Verification items for the finished model (mm, model axes). A direction names the side the tool comes from. Coordinates: 2 decimals unless noted, no trailing zeros. Loops run counter-clockwise (first coordinate to the right, second up) from the corner with the lowest first, then second, coordinate; pieces in that order, holes last. Notation, with made-up numbers: (46.25, 28) -> (63.25, 28) arc R19 ccw to (63.25, 34) -> close; hole circle Ø11 at (57.25, -8.75). An arc over 180 degrees is marked (long way). Answer as a JSON object with one key per item and string values. Group by question number.
Q1. Cross-section at A-A on z = 9.25. Record the boundary of the cut face in (x, y), and give its area (3 significant figures).
Q2. Release check for a two-part mould opening along X. For faces 6 (the cylindrical face through (53.496, 6.926, -4.93)), 7 (the flat face through (27, 1, 0.81)), 8 (the cylindrical face through (65.2, 0.57, 0.41)), 9 (the flat face through (22, 7, 15.82)) record: released by +X, released by -X, zero draft, split by the parting line, or undercut.
Q3. Gauge pin test, flat ends, axial feed: pin 1 Ø3 at (x, y) = (58, 5.5) entering from +Z; pin 2 Ø3 at (x, z) = (47.5, 7.5) entering from -Y; pin 3 Ø3.5 at (x, z) = (25.5, 4.5) entering from +Y. Record the tip position at first contact, or that the pin passes through.
Q4. Cross-section at D-D on x = 18.5. Record the boundary of the cut face in (y, z), and give its area (3 significant figures).
Q5. Cross-section at C-C on z = -5.5. Record the boundary of the cut face in (x, y).
Q6. Scan lines: L1, parallel to X at y = 13, z = 8.25; L2, parallel to Y at x = 5.1, z = 1.5; L3, parallel to X at y = 7.5, z = -1.25. Record each from-to range of solid material in increasing order.
Q7. Set-up check for faces 1 (the cylindrical face through (34.682, 5.914, -4.93)), 2 (the flat face through (58, 12.2, 4)), 3 (the flat face through (50, 2, 4)), 4 (the flat face through (8, 7, 7.92)), 5 (the flat face through (49, 13, 0.81)): record each of +Z, -Z, +X, -X, +Y, -Y from which the full face is reachable in a straight line by a thin tool's end or side.
Q8. Cross-section at B-B on x = 49.55. Record the boundary of the cut face in (y, z).
Autodesk Inventor part; units mm, degrees
ref_plane "YZ Plane" through (0, 0, 0) normal (1, 0, 0) x (0, 1, 0)
ref_plane "XZ Plane" through (0, 0, 0) normal (0, 1, 0) x (-1, 0, 0)
ref_plane "XY Plane" through (0, 0, 0) normal (0, 0, 1) x (1, 0, 0)
sketch "Sketch1" plane through (0, 0, 0) normal (0, 0, 1) x (1, 0, 0)
  line L0 (0, 0) -> (65.8, 0)
  line L1 (65.8, 0) -> (65.8, 14.2)
  line L2 (65.8, 14.2) -> (0, 14.2)
  line L3 (0, 14.2) -> (0, 0)
  dimension "d0" = 65.8
  dimension "d1" = 14.2
extrude "Extrusion1" add sketch "Sketch1" along normal blind 0.81
fillet "Fillet1" radius 2 4 edges at (0, 14.2, 0.405) (65.8, 14.2, 0.405) (65.8, 0, 0.405) (0, 0, 0.405)
sketch "Sketch2" plane through (0, 0, 0.81) normal (0, 0, 1) x (1, 0, 0)
  circle A0 centre (5.1, 7.1) radius 5.1
  line L0 (0, 12.2) -> (0, 2)
  circle A1 centre (60.7, 7.1) radius 5.1
  line L1 (65.8, 2) -> (65.8, 12.2)
  line L2 (5.1, 12.2) -> (60.7, 12.2)
  line L3 (60.7, 2) -> (5.1, 2)
  point P0 (0, 0)
  point P1 (0, 7.1)
  dimension "d5" = 10.2
  dimension "d6" = 10.2
extrude "Extrusion2" add sketch "Sketch2" along normal blind 7.11
sketch "Sketch3" plane through (0, 0, 7.92) normal (0, 0, 1) x (1, 0, 0)
  line L0 (2, 0) -> (63.8, 0)
  line L1 (32.9, 0) -> (32.9, 14.2) construction
  line L2 (63.8, 14.2) -> (2, 14.2)
  circle A0 centre (5.1, 7.1) radius 2.4
  circle A1 centre (60.7, 7.1) radius 2.4
  line L3 (5.1, 7.1) -> (60.7, 7.1) construction
  point P0 (0, 0)
  dimension "d9" = 4.8
  dimension "d10" = 4.8
  dimension "d12" = 27.8
  dimension "d13" = 27.8
  dimension "d14" = 7.1
extrude "Extrusion3" cut sketch "Sketch3" against normal through all
sketch "Sketch4" plane through (0, 0, 7.92) normal (0, 0, 1) x (1, 0, 0)
  line L0 (63.8, 14.2) -> (2, 14.2)
  line L1 (32.9, 14.2) -> (32.9, 0) construction
  line L2 (2, 0) -> (63.8, 0)
  line L3 (31.9, 14.2) -> (33.9, 14.2)
  line L4 (33.9, 14.2) -> (33.9, 0)
  line L5 (33.9, 0) -> (31.9, 0)
  line L6 (31.9, 0) -> (31.9, 14.2)
  line L7 (20.8, 14.2) -> (22.8, 14.2)
  line L8 (22.8, 14.2) -> (22.8, 0)
  line L9 (22.8, 0) -> (20.8, 0)
  line L10 (20.8, 0) -> (20.8, 14.2)
  line L11 (11.7, 0) -> (9.7, 0)
  line L12 (9.7, 0) -> (9.7, 14.2)
  line L13 (9.7, 14.2) -> (11.7, 14.2)
  line L14 (11.7, 14.2) -> (11.7, 0)
  line L15 (43, 14.2) -> (45, 14.2)
  line L16 (45, 14.2) -> (45, 0)
  line L17 (45, 0) -> (43, 0)
  line L18 (43, 0) -> (43, 14.2)
  line L19 (54.1, 0) -> (56.1, 0)
  line L20 (56.1, 0) -> (56.1, 14.2)
  line L21 (56.1, 14.2) -> (54.1, 14.2)
  line L22 (54.1, 14.2) -> (54.1, 0)
  point P0 (0, 0)
  dimension "d17" = 2
  dimension "d18" = 1
  dimension "d19" = 2
  dimension "d20" = 11.1
  dimension "d21" = 11.1
  dimension "d22" = 2
  dimension "d23" = 2
  dimension "d24" = 11.1
  dimension "d25" = 2
  dimension "d26" = 11.1
extrude "Extrusion4" add sketch "Sketch4" along normal mid plane 15.8 contours L20 L2 L22 L0 | L16 L2 L18 L0 | L4 L2 L6 L0 | L8 L2 L10 L0 | L14 L2 L12 L0
fillet "Fillet2" radius 2 10 edges at (10.7, 14.2, 15.82) (21.8, 14.2, 15.82) (32.9, 14.2, 15.82) (44, 14.2, 15.82) (55.1, 14.2, 15.82) (55.1, 0, 15.82) (44, 0, 15.82) (32.9, 0, 15.82) (21.8, 0, 15.82) (10.7, 0, 15.82)
sketch "Sketch5" plane through (0, 0, 0) normal (0, 0, -1) x (-1, 0, 0)
  arc A0 (-65.8, 7.1) -> (-60.7, 2) centre (-60.7, 7.1) ccw
  line L0 (0, 7.1) -> (0, 2)
  line L1 (-65.8, 7.1) -> (0, 7.1) construction
  circle A1 centre (-38.45, 7.1) radius 3.95
  circle A2 centre (-49.55, 7.1) radius 3.95
  circle A3 centre (-27.35, 7.1) radius 3.95
  circle A4 centre (-16.25, 7.1) radius 3.95
  line L2 (-2, 0) -> (-63.8, 0)
  line L3 (-32.9, 0) -> (-32.9, 14.1224) construction
  line L4 (-31.9, 2) -> (-31.9, 12.2)
  point P0 (0, 0)
  dimension "d30" = 7.9
  dimension "d31" = 7.9
  dimension "d32" = 7.9
  dimension "d33" = 7.9
  dimension "d34" = 5.55
  dimension "d35" = 5.55
  dimension "d36" = 11.1
  dimension "d37" = 11.1
extrude "Extrusion5" add sketch "Sketch5" along normal blind 10
properties part number "52160004A"
Computed values:
{
 "1": {"outline": "(9.7, 0) -> (11.7, 0) -> (11.7, 14.2) -> (9.7, 14.2) -> close; (20.8, 0) -> (22.8, 0) -> (22.8, 14.2) -> (20.8, 14.2) -> close; (31.9, 0) -> (33.9, 0) -> (33.9, 14.2) -> (31.9, 14.2) -> close; (43, 0) -> (45, 0) -> (45, 14.2) -> (43, 14.2) -> close; (54.1, 0) -> (56.1, 0) -> (56.1, 14.2) -> (54.1, 14.2) -> close", "area": "142 mm²"},
 "2": {"face 6": "undercut", "face 7": "undercut", "face 8": "released by +X", "face 9": "zero draft"},
 "3": {"pin 1": "stops at z = 7.92", "pin 2": "stops at y = 2", "pin 3": "stops at y = 12.2"},
 "4": {"outline": "(0, 0) -> (3.85, 0) -> (3.85, -10) -> (10.35, -10) -> (10.35, 0) -> (14.2, 0) -> (14.2, 0.81) -> (12.2, 0.81) -> (12.2, 7.92) -> (2, 7.92) -> (2, 0.81) -> (0, 0.81) -> close", "area": "149 mm²"},
 "5": {"outline": "circle Ø7.9 at (16.25, 7.1); circle Ø7.9 at (27.35, 7.1); circle Ø7.9 at (38.45, 7.1); circle Ø7.9 at (49.55, 7.1)"},
 "6": {"L1": "x = 9.7 to 11.7, 20.8 to 22.8, 31.9 to 33.9, 43 to 45, 54.1 to 56.1", "L2": "y = 2 to 4.7, 9.5 to 12.2", "L3": "x = 12.32 to 20.18, 23.42 to 31.28, 34.52 to 42.38, 45.62 to 53.48"},
 "7": {"face 1": "-Z", "face 2": "+Z, +X, +Y", "face 3": "+Z, -Y", "face 4": "+Z, -X, +Y, -Y", "face 5": "+Z, +Y"},
 "8": {"outline": "(0, 0) -> (3.15, 0) -> (3.15, -10) -> (11.05, -10) -> (11.05, 0) -> (14.2, 0) -> (14.2, 0.81) -> (12.2, 0.81) -> (12.2, 7.92) -> (2, 7.92) -> (2, 0.81) -> (0, 0.81) -> close"}
}
